For this review, take the finished solid that the model builds, in its own axes (mm). A direction names the side the tool comes from. Round coordinates to 2 decimals unless told otherwise and drop trailing zeros. Order: outer loops, then holes, each group sorted by start corner. A loop starts at its lowest first (then second) coordinate and runs counter-clockwise, first axis right, second up. Notation, with made-up numbers: (-7, -31.5) -> (28, -31.5) arc R15 cw to (28, -2.5) -> close; hole circle Ø4 at (48.25, -25). An arc over 180 degrees is marked (long way). Use a Markdown table: item, result. Add a question column.
1) Consider section A-A (x = 37). State the section outline as (y, z) points, plus the area to 3 significant figures.
2) Clearance check with flat-ended pins moving along their axes: P1, Ø2.5, axis at x = -6, y = 8.5, coming from the -Z side; P2, Ø3.5, axis at x = -5, z = 7, coming from the +Y side; P3, Ø1, axis at x = 34.5, z = 9.5, coming from the -Y side; P4, Ø2, axis at x = 18, y = -15.5, coming from the +Z side. State where each tip first meets the part, or that it passes through.
3) Consider section C-C (z = 5). State the section outline as (x, y) points, plus the area to 3 significant figures.
4) Consider section B-B (y = -30.5). State the section outline as (x, z) points.
5) Consider section D-D (x = -4). State the section outline as (y, z) points.
6) Wall thickness on line 1 along X through (y, z) = (7.5, 8.75); line 2 along X through (y, z) = (-8.5, 3.25); line 3 along Y through (x, z) = (-7, 4.5): over which ranges is each line inside the solid? List them lowest first. Write a range as [from, to].
7) Draft analysis for pull direction X (two halves, no side actions). For faces 1 (the face through (2, 5, 15)), 2 (the face through (-56.28, -20.42, 13.5)), 3 (the face through (-52.44, -25, 9)), state which applies: pulls with the +X half, pulls with the -X half, needs draft (parallel to the pull), parting line crosses it, or undercut.
8) Machinability: for faces 4 (the face through (1, -25, 3)), 5 (the face through (2, 9, 2)), 6 (the face through (3, 10, 14)), which of the approach directions +Z, -Z, +X, -X, +Y, -Y give a long, thin tool a straight path to every point of the face, cutting with its end or side? Answer none if there is none.
```python
from build123d import *

# Parameters (mm, degrees)
F0_W     = 107.7930156246
F0_H     = 50
F1_DEPTH = 3
F2_DEPTH = 15
F3_R     = 5
F3_2_R   = 5
F5_W     = 52
F5_H     = 11
F6_DEPTH = 3


with BuildPart() as f1:
    # F0 (on Top) → F1 (new body)
    with BuildSketch(Plane.XY):
        Polygon((-57.7105433475, 0), (-57.7105433475, -50), (-52.4395332623, -50), (-52.4395332623, 0), (55.3534823623, 0), (55.3534823623, -50), (62.2894566525, -50), (62.2894566525, 0), (62.2894566525, 10), (-57.7105433475, 10), align=None)
        with Locations((1.45697455, -25)):
            Rectangle(F0_W, F0_H)
    extrude(amount=F1_DEPTH)

    # F3#2
    f3_2_edges = [f1.edges().sort_by_distance(p)[0] for p in [
        (-57.710543, -50, 1.5),
        (62.289457, -50, 1.5),
    ]]
    fillet(f3_2_edges, radius=F3_2_R)


with BuildPart() as f2:
    # F0 (on Top) → F2 (new body)
    with BuildSketch(Plane.XY):
        Polygon((-57.7105433475, 0), (-57.7105433475, -50), (-52.4395332623, -50), (-52.4395332623, 0), (55.3534823623, 0), (55.3534823623, -50), (62.2894566525, -50), (62.2894566525, 0), (62.2894566525, 10), (-57.7105433475, 10), align=None)
    extrude(amount=F2_DEPTH)

    # F3
    f3_edges = [f2.edges().sort_by_distance(p)[0] for p in [
        (-57.710543, -20, 15),
        (62.289457, -20, 15),
    ]]
    fillet(f3_edges, radius=F3_R)


with BuildPart() as f1_1:
    add(f1.part)

    # F4: union F2
    add(f2.part)

    # F5 (on face) → F6 (cut)
    with BuildSketch(Plane(origin=(0, 10, 0), x_dir=(-1, 0, 0), z_dir=(0, 1, 0))):
        with Locations((-1.9977902994, 7.5)):
            Rectangle(F5_W, F5_H)
    extrude(amount=-F6_DEPTH, mode=Mode.SUBTRACT)


solid = f1_1.part
```
Results list:
| question | item | result |
|---|---|---|
| 1 | outline | (-50, 0) -> (10, 0) -> (10, 15) -> (0, 15) -> (0, 3) -> (-50, 3) -> close |
| 1 | area | 300 mm2 |
| 2 | P1 | z = 0 |
| 2 | P2 | y = 7 |
| 2 | P3 | y = 0 |
| 2 | P4 | z = 3 |
| 3 | outline | (-57.71, -50) -> (-52.44, -50) -> (-52.44, 0) -> (55.35, 0) -> (55.35, -50) -> (62.29, -50) -> (62.29, 10) -> (28, 10) -> (28, 7) -> (-24, 7) -> (-24, 10) -> (-57.71, 10) -> close |
| 3 | area | 1,650 mm2 |
| 4 | outline | (-57.71, 0) -> (62.29, 0) -> (62.29, 10) arc R5 ccw to (57.29, 15) -> (55.35, 15) -> (55.35, 3) -> (-52.44, 3) -> (-52.44, 15) -> (-52.71, 15) arc R5 ccw to (-57.71, 10) -> close |
| 5 | outline | (-50, 0) -> (10, 0) -> (10, 2) -> (7, 2) -> (7, 13) -> (10, 13) -> (10, 15) -> (0, 15) -> (0, 3) -> (-50, 3) -> close |
| 6 | line 1 | [-57.71, -24], [28, 62.29] |
| 6 | line 2 | [-57.71, -52.44], [55.35, 62.29] |
| 6 | line 3 | [0, 7] |
| 7 | face 1 | needs draft |
| 7 | face 2 | pulls with the -X half |
| 7 | face 3 | undercut |
| 8 | face 4 | +Z, -Y |
| 8 | face 5 | +Y |
| 8 | face 6 | +Z, -Z, +X, -X, +Y |
